Answer from the drawing. Dimensions are ordinates in mm from the lowest x, y and z of the part. A direction names the side the tool comes from. Round coordinates to 2 decimals unless told otherwise and drop trailing zeros. Write each loop counter-clockwise with the first axis right and the second up, starting at its lowest first coordinate (ties: lowest second). Pieces come first, ordered by that corner, then holes. Notation, with made-up numbers: (9.25, 46.25) - (44.25, 46.25) arc R14 cw to (44.25, 64.25) - close; hole circle Ø3 at (42.25, 86.5). An arc over 180 degrees is marked (long way). Write item = value, one per line. Start each with the question number.
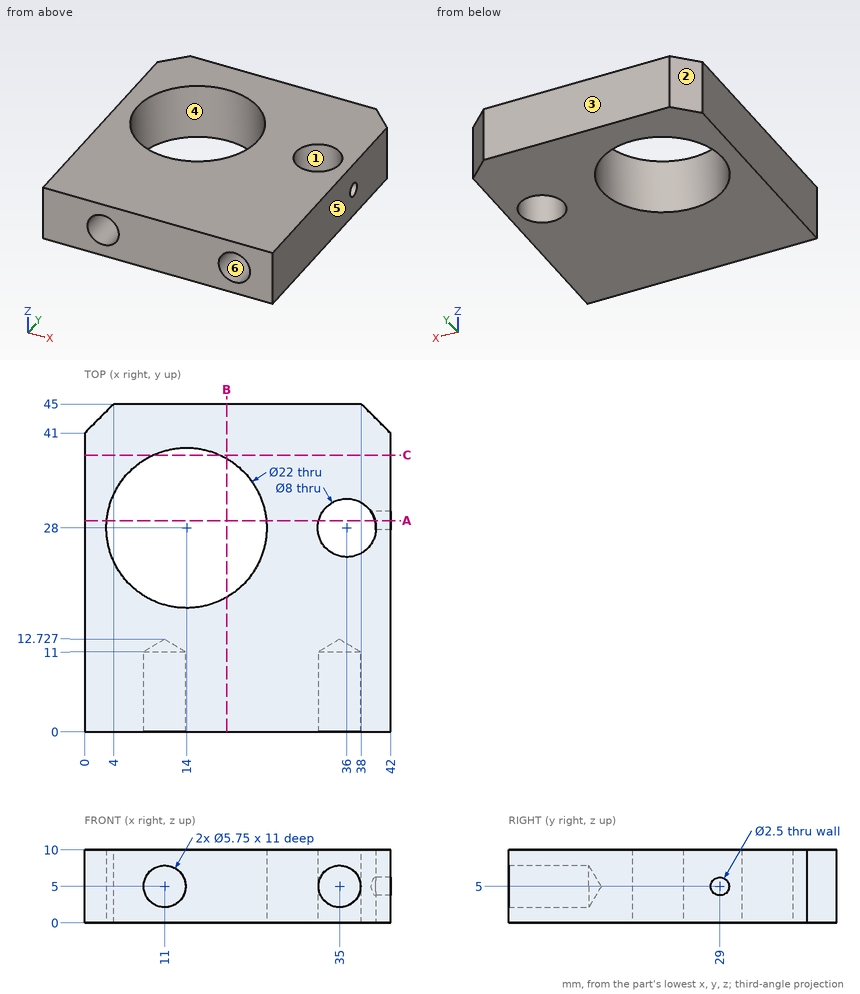
1. Find section C-C on y = 38. Give the vertices of the cut face in (x, z), plus the area to 3 significant figures.
2. Find section A-A on y = 29. Give the number of separate pieces and of enclosed holes in the cut face, plus the area to 3 significant figures.
3. Find section B-B on x = 19.5. Give the vertices of the cut face in (y, z).
4. Which of the six approach directions +Z, -Z, +X, -X, +Y, -Y give full straight-line access (tool end or side, diameter ignored) to the marked faces 5 and 6?
5. Each of these flat-tipped pins is pushed along its axis until it touches: pin 1 (20 mm diameter, centred on x = 14, y = 28, fed in from +Z); pin 2 (2 mm diameter, centred on x = 36, z = 4, fed in from -Y). Where does it stop, or does it pass through?
6. For a pull along X with two mould halves and no side action, classify the marked faces 1, 2, 3 and 4 as released by +X, released by -X, zero draft, split by the parting line, or undercut.
7. Consider line 1 (Y direction, x = 14.5, z = 9.25); line 2 (Z direction, x = 35, y = 2.5) (1 decimal); line 3 (X direction, y = 2, z = 2.5). Determine where each line is inside the solid, lowest interval first.
Answer key:
q1.outline = (0, 0) - (9.42, 0) - (9.42, 10) - (0, 10) - close; (18.58, 0) - (42, 0) - (42, 10) - (18.58, 10) - close
q1.area = 328 mm²
q2.separate_pieces = 4
q2.enclosed_holes = 0
q2.area = 118 mm²
q3.outline = (0, 0) - (18.47, 0) - (18.47, 10) - (0, 10) - close; (37.53, 0) - (45, 0) - (45, 10) - (37.53, 10) - close
q4.face_5 = +Z, -Z, +X, +Y, -Y
q4.face_6 = -Y
q5.pin_1 = through
q5.pin_2 = 11.28
q6.face_1 = undercut
q6.face_2 = released by -X
q6.face_3 = zero draft
q6.face_4 = undercut
q7.line_1 = 0 to 17.01, 38.99 to 45
q7.line_2 = 0 to 2.1, 7.9 to 10
q7.line_3 = 0 to 9.58, 12.42 to 33.58, 36.42 to 42
